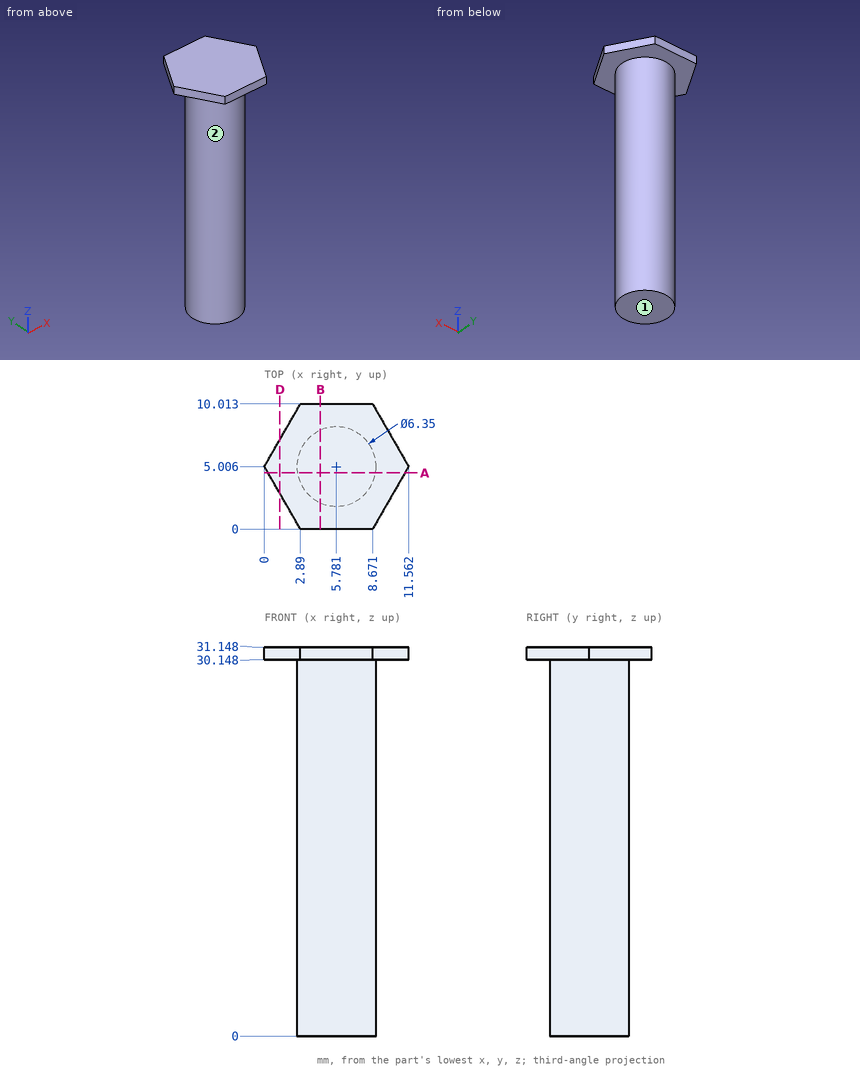
Geometry: see drawing. Coordinates: mm, zero at the bounding-box minimum. A direction names the side the tool comes from. Coordinates: 2 decimals unless noted, no trailing zeros. Write each loop counter-clockwise with the first axis right and the second up, starting at its lowest first coordinate (ties: lowest second). Pieces come first, ordered by that corner, then holes. Notation, with made-up numbers: M -29,71 L -13,71 A23 cw -13,84 Z; hole C 16,56 d8. An arc over 180 degrees is marked long. Answer as a JSON object with one key per item and string values.
1. Contact query for flat-ended pins moving along their axis: P1, Ø1.5, axis at x = 1.5, z = 10, coming from the +Y side; P2, Ø1, axis at y = 6.5, z = 7.5, coming from the +X side; P3, Ø6, axis at y = 3.5, z = 20, coming from the -X side; P4, Ø4, axis at x = 6, y = 4, coming from the -Z side. Output: stop coordinate, or through.
Evaluation:
{"P1": "through", "P2": "x = 8.8", "P3": "x = 2.61", "P4": "z = 0"}
2. Access query for the marked faces 1 and 2. Directions: +Z, -Z, +X, -X, +Y, -Y. A direction counts if a zero-diameter tool reaches every point of the face in a straight line with its end or side. Return the directions, or none.
Evaluation:
{"face 1": "-Z, +X, -X, +Y, -Y", "face 2": "-Z"}
3. Ray query, L1, parallel to Y at x = 6, z = 9; L2, parallel to X at y = 4, z = 17; L3, parallel to X at y = 3, z = 14. Return the intervals inside material, ascending.
Evaluation:
{"L1": "1.84 to 8.17", "L2": "2.77 to 8.79", "L3": "3.32 to 8.24"}
4. Cut plane D-D on x = 1.25. Output: boundary loops of the cut face in (y, z).
Evaluation:
{"outline": "M 2.84,30.15 L 7.17,30.15 L 7.17,31.15 L 2.84,31.15 Z"}
5. Cut plane A-A on y = 4.5. Output: boundary loops of the cut face in (x, z) (1 decimal), plus the area to 3 significant figures.
Evaluation:
{"outline": "M 0.3,30.1 L 2.6,30.1 L 2.6,0 L 8.9,0 L 8.9,30.1 L 11.3,30.1 L 11.3,31.1 L 0.3,31.1 Z", "area": "200 mm^2"}
6. Cut plane B-B on x = 4.5. Output: boundary loops of the cut face in (y, z), plus the area to 3 significant figures.
Evaluation:
{"outline": "M 0,30.15 L 2.1,30.15 L 2.1,0 L 7.91,0 L 7.91,30.15 L 10.01,30.15 L 10.01,31.15 L 0,31.15 Z", "area": "185 mm^2"}
